Verification items for the finished model (mm, model axes). Face numbers are marked on the shaded views. A direction names the side the tool comes from. Round coordinates to 2 decimals unless told otherwise and drop trailing zeros. Order: outer loops, then holes, each group sorted by start corner. A loop starts at its lowest first (then second) coordinate and runs counter-clockwise, first axis right, second up. Notation, with made-up numbers: M 24,58.5 L 66,58.5 A19 ccw 66,89.5 Z; hole C -29,23.25 d10. An arc over 180 degrees is marked long. Return JSON: item names as keys, results as strings. Group by question number.
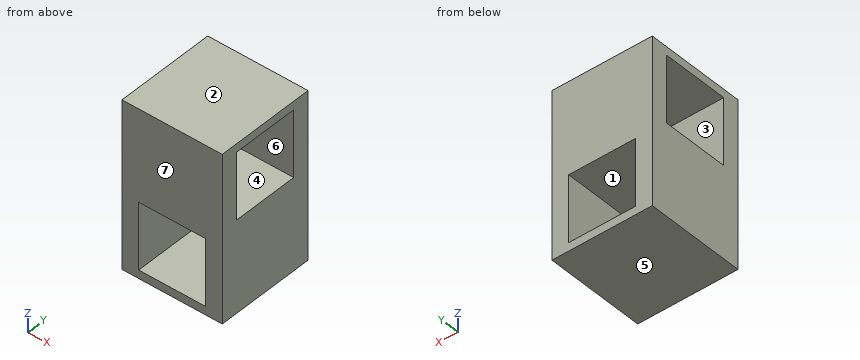
from build123d import *

# Parameters (mm, degrees)
SKETCH1_W           = 30
SKETCH1_H           = 30
BOSS_EXTRUDE1_DEPTH = 50
SKETCH3_W           = 20
SKETCH3_H           = 20
CUT_EXTRUDE1_DEPTH  = 61.207972894
SKETCH4_W           = 20
SKETCH4_H           = 20
CUT_EXTRUDE2_DEPTH  = 61.207972894


with BuildPart() as part:
    # Sketch1 → Boss-Extrude1 (new body)
    with BuildSketch(Plane.XY):
        Rectangle(SKETCH1_W, SKETCH1_H)
    extrude(amount=BOSS_EXTRUDE1_DEPTH)

    # Sketch3 → Cut-Extrude1 (cut, through all)
    with BuildSketch(Plane.ZY.offset(15)):
        with Locations((37.5, 0)):
            Rectangle(SKETCH3_W, SKETCH3_H)
    extrude(amount=-CUT_EXTRUDE1_DEPTH, mode=Mode.SUBTRACT)

    # Sketch4 → Cut-Extrude2 (cut, through all)
    with BuildSketch(Plane(origin=(0, 15, 0), x_dir=(1, 0, 0), z_dir=(0, 1, 0))):
        with Locations((0, -12.5)):
            Rectangle(SKETCH4_W, SKETCH4_H)
    extrude(amount=-CUT_EXTRUDE2_DEPTH, mode=Mode.SUBTRACT)


solid = part.part
1. Draft check along Y on the marked faces 4, 5, 6 and 7. Enter one of: +Y half, -Y half, draft (parallel to the pull), parting line (faces both ways), or undercut.
2. Access from +Z, -Z, +X, -X, +Y, -Y to the whole of each face (thin tool, end or side, straight path). Record for the marked faces 1, 2 and 3.
3. Thickness scan on line 1 along Z through (x, y) = (-4.75, 7); line 2 along Z through (x, y) = (11, -6.5); line 3 along X through (y, z) = (9.5, 16.5). Record the ranges inside material, lowest first. Write a range as from..to.
4. Cross-section at C-C (y = 1.5). Enter the section's corners in (x, z).
5. Cross-section at B-B (z = 5). Enter the section's corners in (x, y).
6. Cross-section at A-A (x = 4.25). Enter the section's corners in (y, z), plus the area to 3 significant figures.
Computed:
{
 "1": {"face 4": "undercut", "face 5": "draft", "face 6": "undercut", "face 7": "-Y half"},
 "2": {"face 1": "+Y, -Y", "face 2": "+Z, +X, -X, +Y, -Y", "face 3": "+X, -X"},
 "3": {"line 1": "z = 0..2.5, 22.5..27.5, 47.5..50", "line 2": "z = 0..27.5, 47.5..50", "line 3": "x = -15..-10, 10..15"},
 "4": {"outline": "M -15,0 L 15,0 L 15,27.5 L -15,27.5 Z; M -15,47.5 L 15,47.5 L 15,50 L -15,50 Z; hole M -10,2.5 L 10,2.5 L 10,22.5 L -10,22.5 Z"},
 "5": {"outline": "M -15,-15 L -10,-15 L -10,15 L -15,15 Z; M 10,-15 L 15,-15 L 15,15 L 10,15 Z"},
 "6": {"outline": "M -15,0 L 15,0 L 15,2.5 L -15,2.5 Z; M -15,22.5 L 15,22.5 L 15,50 L -15,50 Z; hole M -10,27.5 L 10,27.5 L 10,47.5 L -10,47.5 Z", "area": "500 mm²"}
}
